Could you check a few things on this model? Use its own coordinates, in mm. Round coordinates to 2 decimals unless told otherwise and drop trailing zeros. Loops run counter-clockwise (first coordinate to the right, second up) from the corner with the lowest first, then second, coordinate; pieces in that order, holes last. Notation, with made-up numbers: (-16.75, 41) - (2.25, 41) arc R19 cw to (2.25, 58) - close; hole circle Ø7 at (34.5, 14). An arc over 180 degrees is marked (long way). Use one line per item in the form item = value.
```python
from build123d import *

# Parameters (mm, degrees)
F0_W     = 110
F0_H     = 60
F1_DEPTH = 2
F2_R     = 5
F3_W     = 3
F3_H     = 3
F4_DEPTH = 25
F5_R     = 1
F6_R     = 1.75
F7_DEPTH = 25


with BuildPart() as f1:
    # F0 (on Top) → F1 (new body)
    with BuildSketch(Plane.XY):
        Rectangle(F0_W, F0_H)
    extrude(amount=F1_DEPTH)

    # F2
    f2_edges = [f1.edges().sort_by_distance(p)[0] for p in [
        (55, -30, 1),
        (55, 30, 1),
        (-55, 30, 1),
        (-55, -30, 1),
    ]]
    fillet(f2_edges, radius=F2_R)

    # F3 (on face) → F4 (cut)
    with BuildSketch(Plane.XY.offset(2)):
        with Locations((0, 28.5)):
            Rectangle(F3_W, F3_H)
    extrude(amount=-F4_DEPTH, mode=Mode.SUBTRACT)

    # F5
    f5_edges = [f1.edges().sort_by_distance(p)[0] for p in [
        (-1.5, 30, 1),
        (-1.5, 27, 1),
        (1.5, 27, 1),
        (1.5, 30, 1),
    ]]
    fillet(f5_edges, radius=F5_R)

    # F6 (on face) → F7 (cut)
    with BuildSketch(Plane.XY.offset(2)):
        Circle(F6_R)
    extrude(amount=-F7_DEPTH, mode=Mode.SUBTRACT)


solid = f1.part
```
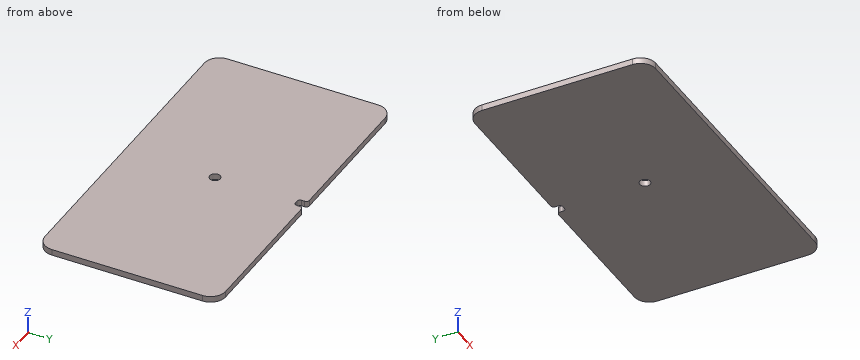
1. If we section it at A-A, the plane y = 0: Write out the boundary of the cut face in (x, z), plus the area to 3 significant figures.
Solution:
outline = (-55, 0) - (-1.75, 0) - (-1.75, 2) - (-55, 2) - close; (1.75, 0) - (55, 0) - (55, 2) - (1.75, 2) - close
area = 213 mm^2
2. Please list where this line runs through material, in increasing order: line 1 along Y through (x, z) = (0, 1.45).
Solution:
line_1 = -30 to -1.75, 1.75 to 27
3. For P1, Ø0.8, axis at x = 0, z = 1.5, coming from the +Y side; P2, Ø2, axis at x = 3, y = -0.5, coming from the -Z side; P3, Ø1.1, axis at y = 28.5, z = 0.5, coming from the +X side, each with a flat end and sliding along its axis, tell me the tip position at first contact or that it passes through.
Solution:
P1 = 27
P2 = 0
P3 = 54.04
